Work out the finished part from the listing and answer in its coordinate system (mm). A direction names the side the tool comes from. Coordinates: 2 decimals unless noted, no trailing zeros. Write each loop counter-clockwise with the first axis right and the second up, starting at its lowest first coordinate (ties: lowest second). Pieces come first, ordered by that corner, then holes. Notation, with made-up numbers: (42, 41) - (66, 41) arc R36 cw to (66, 75) - close; hole circle Ø4 at (11.5, -33). An arc over 180 degrees is marked (long way). Use a Markdown table: item, result. Add a question column.
(1) A tool of negligible diameter and unlimited length cuts with its end or side. For faces 4 (the face through (21.11, 2.48, 7.41)), 5 (the face through (0, 24.75, 0)), 6 (the face through (0, 103.75, 0)), 7 (the face through (-21.114, 6.184, -6.992)), from which of +Z, -Z, +X, -X, +Y, -Y can it reach the whole face along a straight path? Write none if from no direction.
(2) Given pin 1 Ø4 at (x, z) = (-13, -1) entering from +Y; pin 2 Ø2 at (y, z) = (1.55, -8) entering from +X; pin 3 Ø1.5 at (x, z) = (17, -5.5) entering from -Y, each flat-ended and moving along its own axis, determine where each tip first touches the part or whether it passes through.
(3) For a pull along Y with two mould halves and no side action, classify faces 1 (the face through (20.1, 12, 0)), 2 (the face through (21.114, 20.696, 0.238)), 3 (the face through (21.11, 126.25, 0.08)) as released by +Y, released by -Y, zero draft, split by the parting line, or undercut.
(4) The part is cut by section A-A, the plane y = 10. Give the vertices of the cut face in (x, z), then the cut area to 3 significant figures.
(5) Find the intervals of material crossed by line 1 (Y direction, x = -21.45, z = -7.5); line 2 (Z direction, x = -10, y = 13); line 3 (X direction, y = 18, z = -5), in increasing order. Write a range as from..to.
(6) The part is cut by section B-B, the plane x = 10. Give the vertices of the cut face in (y, z), then the cut area to 3 significant figures.
Autodesk Inventor part; units mm, degrees
ref_plane "РабПлоскость5" through (0, 64.25, 0) normal (0, 1, 0) x (1, 0, 0)
ref_plane "РабПлоскость1" through (0, 48, 0) normal (0, 1, 0) x (1, 0, 0)
ref_plane "YZ Plane" through (0, 0, 0) normal (1, 0, 0) x (0, 1, 0)
sketch "Эскиз2" plane through (0, 0, 0) normal (0, 1, 0) x (-1, 0, 0)
  line L0 (20.1, -10) -> (-20.1, -10)
  line L1 (-20.1, -10) -> (-20.1, 10)
  line L2 (-20.1, 10) -> (20.1, 10)
  line L3 (20.1, 10) -> (20.1, -10)
  line L4 (20.1, -10) -> (-20.1, 10) construction
  line L5 (-20.1, -10) -> (20.1, 10) construction
  line L6 (22.1, 12) -> (-22.1, 12)
  line L7 (-22.1, 12) -> (-22.1, -12)
  line L8 (-22.1, -12) -> (22.1, -12)
  line L9 (22.1, -12) -> (22.1, 12)
  line L10 (22.1, 12) -> (-22.1, -12) construction
  line L11 (-22.1, 12) -> (22.1, -12) construction
  point P0 (0, 0)
  dimension "d5" = 40.2
  dimension "d6" = 20
  dimension "d7" = 2
  dimension "d8" = 2
extrude "Выдавливание1" add sketch "Эскиз2" along normal blind 24.75
sketch "Эскиз4" plane through (22.1, 0, 12) normal (1, 0, 0) x (0, 0, -1)
  line L0 (0, 0) -> (24, 0)
  line L1 (24, 0) -> (24, 24.75)
  line L2 (0, 24.75) -> (24, 24.75)
  line L3 (0, 0) -> (0, 24.75)
  line L4 (22, 24.75) -> (2, 24.75)
  line L5 (12, 24.75) -> (12, 1.55) construction
  line L6 (12, 1.55) -> (20, 1.55) construction
  circle A0 centre (20, 1.55) radius 1.1
  line L7 (12, 14.77) -> (19, 14.77) construction
  circle A1 centre (19, 14.77) radius 1.1
  circle A2 centre (12, 21.77) radius 1.1
  circle A3 centre (4, 1.55) radius 1.1
  line L8 (12, 14.77) -> (5, 14.77) construction
  circle A4 centre (5, 14.77) radius 1.1
  line L9 (12, 1.55) -> (4, 1.55) construction
  point P0 (12, 0)
  dimension "d13" = 23.2
  dimension "d14" = 8
  dimension "d15" = 2.2
  dimension "d16" = 7
  dimension "d17" = 13.22
  dimension "d18" = 7
extrude "Выдавливание3" cut sketch "Эскиз4" against normal blind 2 contours A0 | A1 | A2 | A3 | A4
sketch "Эскиз5" plane through (-22.1, 0, -12) normal (-1, 0, 0) x (0, 0, 1)
  line L0 (0, 0) -> (24, 0)
  line L1 (24, 0) -> (24, 24.75)
  line L2 (0, 24.75) -> (24, 24.75)
  line L3 (0, 0) -> (0, 24.75)
  line L4 (24, 24.75) -> (0, 24.75)
  line L5 (12, 24.75) -> (12, 5.2772) construction
  circle A0 centre (19.5, 22.16) radius 1.1
  line L6 (19.5, 22.16) -> (12, 22.16) construction
  circle A1 centre (4.5, 22.16) radius 1.1
  circle A2 centre (19.5, 7.16) radius 1.1
  circle A3 centre (4.5, 7.16) radius 1.1
  point P0 (12, 0)
  dimension "d21" = 2.59
  dimension "d22" = 7.5
  dimension "d23" = 2.2
  dimension "d26" = 15
  dimension "d29" = 15
extrude "Выдавливание4" cut sketch "Эскиз5" against normal blind 2 contours A0 | A1 | A2 | A3
sketch "Эскиз3" plane through (0, 24.75, 0) normal (0, 1, 0) x (1, 0, 0)
  line L0 (-22.1, -12) -> (22.1, -12)
  line L1 (22.1, -12) -> (-22.1, -12)
  line L2 (-22.1, -12) -> (-22.1, 12)
  line L3 (-22.1, 12) -> (22.1, 12)
  line L4 (22.1, 12) -> (22.1, -12)
  point P0 (0, 0)
extrude "Выдавливание2" add sketch "Эскиз3" along normal blind 2
ref_plane "РабПлоскость3" through (-22.1, 26.75, -12) normal (0, 1, 0) x (1, 0, 0)
sketch "Эскиз7" plane through (0, 26.75, 0) normal (0, 1, 0) x (1, 0, 0)
  line L0 (22.1, -12) -> (22.1, 12)
  line L1 (-22.1, 12) -> (-22.1, -12)
  line L2 (22.1, -12) -> (-22.1, -12)
  line L3 (-22.1, -12) -> (-22.1, 12)
  line L4 (-22.1, 12) -> (22.1, 12)
  line L5 (22.1, 12) -> (22.1, -12)
  point P0 (0, 0)
extrude "Выдавливание5" add sketch "Эскиз7" along normal blind 75
ref_plane "РабПлоскость5" through (0, 64.25, 0) normal (0, 1, 0) x (1, 0, 0)
mirror "Зеркальное отражение2" about plane through (0, 64.25, 0) normal (0, 1, 0) of "Выдавливание3", "Выдавливание1", "Выдавливание4", "Выдавливание2"
sketch "Эскиз9" plane through (22.1, 0, 12) normal (1, 0, 0) x (0, 0, -1)
  circle A0 centre (20, 126.95) radius 1.1 construction
  circle A1 centre (4, 126.95) radius 1.1 construction
  circle A2 centre (19, 113.73) radius 1.1 construction
  circle A3 centre (5, 113.73) radius 1.1 construction
  circle A4 centre (12, 106.73) radius 1.1 construction
  circle A5 centre (20, 1.55) radius 1.1 construction
  circle A6 centre (4, 1.55) radius 1.1 construction
  circle A7 centre (19, 14.77) radius 1.1 construction
  circle A8 centre (5, 14.77) radius 1.1 construction
  circle A9 centre (12, 21.77) radius 1.1 construction
  line L0 (0, 0) -> (24, 0) construction
  line L1 (24, 0) -> (24, 128.5) construction
  line L2 (0, 128.5) -> (24, 128.5) construction
  line L3 (0, 0) -> (0, 128.5) construction
  line L4 (0, 0) -> (0, 128.5) construction
  line L5 (0, 64.25) -> (24, 64.25) construction
  circle A10 centre (12, -5.25) radius 7.5
  line L6 (12, -5.25) -> (12, 0) construction
  circle A11 centre (12, 133.75) radius 7.5
  dimension "d46" = 15
  dimension "d47" = 5.25
extrude "Выдавливание6" cut sketch "Эскиз9" against normal up to surface (44.2 mm away)
sketch "Эскиз6" plane through (0, 48, 0) normal (0, 1, 0) x (1, 0, 0)
  line L0 (-12, -22.1) -> (12, -22.1)
  line L1 (12, -22.1) -> (12, 22.1)
  line L2 (12, 22.1) -> (-12, 22.1)
  line L3 (-12, 22.1) -> (-12, -22.1)
  line L4 (-12, -22.1) -> (12, 22.1) construction
  line L5 (12, -22.1) -> (-12, 22.1) construction
  point P0 (0, 0)
  dimension "d35" = 44.2
  dimension "d36" = 24
equation "\"d48\" = d46"
properties part number "мотор_локтя_2.1-кисти_1"
Model answer:
| question | item | result |
|---|---|---|
| 1 | face 4 | +X |
| 1 | face 5 | -Y |
| 1 | face 6 | +Y |
| 1 | face 7 | -X |
| 2 | pin 1 | y = 103.75 |
| 2 | pin 2 | x = -20.1 |
| 2 | pin 3 | y = 24.75 |
| 3 | face 1 | zero draft |
| 3 | face 2 | undercut |
| 3 | face 3 | released by +Y |
| 4 | outline | (-22.1, -12) - (22.1, -12) - (22.1, 12) - (-22.1, 12) - close; hole (-20.1, -10) - (20.1, -10) - (20.1, 10) - (-20.1, 10) - close |
| 4 | area | 257 mm^2 |
| 5 | line 1 | 0..6.06, 8.26..21.06, 23.26..105.24, 107.44..120.24, 122.44..128.5 |
| 5 | line 2 | -12..-10, 10..12 |
| 5 | line 3 | -22.1..-20.1, 20.1..22.1 |
| 6 | outline | (0, -12) - (128.5, -12) - (128.5, -10) - (103.75, -10) - (103.75, 10) - (128.5, 10) - (128.5, 12) - (0, 12) - (0, 10) - (24.75, 10) - (24.75, -10) - (0, -10) - close |
| 6 | area | 2,090 mm^2 |
